Work out the finished part from the listing and answer in its coordinate system (mm). Coordinates: 2 decimals unless noted, no trailing zeros.
1. The part is cut by section A-A, the plane z = -1.6. Count the separate pieces of the cut face and the enclosed holes in it, then the cut area to 3 significant figures.
2. Flat-ended cylindrical pins translate along their axes: pin 1 Ø10.5 at (x, y) = (60, 0) entering from +Z; pin 2 Ø1 at (x, z) = (-4.5, -0.5) entering from +Y; pin 3 Ø5 at (x, y) = (-32.63, 15.21) entering from -Z; pin 4 Ø1 at (x, z) = (46, -2) entering from -Y. Find the tip coordinate at first contact, or state that the pin passes through.
3. Find the intervals of material crossed by probe 1 along X at (y, z) = (-2.5, -2); probe 2 along X at (y, z) = (3.5, -0.2); probe 3 along Y at (x, z) = (-33, -1.8), in increasing order.
```python
from build123d import *

# Parameters (mm, degrees)
EXTRUDE_1_DEPTH     = 3
SKETCH_2_R          = 4
SKETCH_2_R_2        = 6
CUT_EXTRUDE_1_DEPTH = 5
CUT_EXTRUDE_START   = -10
CUT_EXTRUDE_2_DEPTH = 10
FILLET_1_R          = 2
EXTRUDE_START       = -3
EXTRUDE_2_DEPTH     = 3
FILLET_3_R          = 2
EXTRUDE_START_2     = 0.25
SKETCH_6_R          = 8
EXTRUDE_3_DEPTH     = 0.25
SKETCH_7_R          = 7
SKETCH_7_R_2        = 5
CUT_EXTRUDE_4_DEPTH = 1
SKETCH_4_R          = 86.502313977
CUT_EXTRUDE_5_DEPTH = 11
FILLET_5_R          = 5
FILLET_6_R          = 1
SKETCH_8_R          = 14.07038583
CUT_EXTRUDE_6_DEPTH = 0.25


# Some blends are built 0.0001 mm under size
with BuildPart() as part:
    # 草图1 → 凸台-拉伸1 (new body)
    with BuildSketch(Plane.XY):
        with BuildLine():
            Line((60.533333333, -7.982202425), (0.8, -11.973303638))
            ThreePointArc((0.8, -11.973303638), (-2.939445104, -11.634417153), (-6.391104371, -10.156465178))
            Line((-6.391104371, -10.156465178), (-36.621520565, 8.866466686))
            ThreePointArc((-36.621520565, 8.866466686), (-39.424388736, 18.383894386), (-30.331967202, 22.3544574))
            Line((-30.331967202, 22.3544574), (-0.067539503, 12.626398572))
            ThreePointArc((-0.067539503, 12.626398572), (2.297970236, 12.022555106), (4.719428847, 11.711425782))
            Line((4.719428847, 11.711425782), (60.533333333, 7.982202425))
            ThreePointArc((60.533333333, 7.982202425), (68, 0), (60.533333333, -7.982202425))
        make_face()
    extrude(amount=EXTRUDE_1_DEPTH)

    # 草图2 → 切除-拉伸1 (cut)
    with BuildSketch(Plane.XY.offset(3)):
        with Locations((-32.627080333, 15.214257423)):
            Circle(SKETCH_2_R)
        with Locations((60, 0)):
            Circle(SKETCH_2_R)
        Circle(SKETCH_2_R_2)
    extrude(amount=-CUT_EXTRUDE_1_DEPTH, mode=Mode.SUBTRACT)

    # 草图3 → 切除-拉伸2 (cut)
    with BuildSketch(Plane.XY.offset(3).offset(CUT_EXTRUDE_START)):
        with BuildLine():
            Line((28.230392562, -4.127155499), (29.041000535, 4.072994476))
            Line((29.041000535, 4.072994476), (10.769185117, 5.293831496))
            ThreePointArc((10.769185117, 5.293831496), (11.688246691, 2.71751528), (12, 0))
            ThreePointArc((12, 0), (11.688246691, -2.71751528), (10.769185117, -5.293831496))
            Line((10.769185117, -5.293831496), (28.230392562, -4.127155499))
        make_face()
        with BuildLine():
            ThreePointArc((-11.991309043, 0.456626154), (-10.875693444, 5.071419141), (-8.057660805, 8.892362024))
            Line((-8.057660805, 8.892362024), (-24.425138032, 14.153448832))
            ThreePointArc((-24.425138032, 14.153448832), (-25.131680833, 11.719095235), (-26.54234692, 9.613079718))
            Line((-26.54234692, 9.613079718), (-11.991309043, 0.456626154))
        make_face()
        with BuildLine():
            Line((52.404599069, 2.511948386), (35.030683756, 3.672791932))
            Line((35.030683756, 3.672791932), (34.299724154, -3.721631224))
            Line((34.299724154, -3.721631224), (52.404599069, -2.511948386))
            ThreePointArc((52.404599069, -2.511948386), (52, 0), (52.404599069, 2.511948386))
        make_face()
    extrude(amount=CUT_EXTRUDE_2_DEPTH, mode=Mode.SUBTRACT)

    # 圆角1
    fillet_1_edges = [part.edges().sort_by_distance(p)[0] for p in [
        (52.404599069, 2.511948386, 1.5),
        (52.404599069, -2.511948386, 1.5),
        (34.299724154, -3.721631224, 1.5),
        (35.030683756, 3.672791932, 1.5),
        (-26.54234692, 9.613079718, 1.5),
        (-24.425138032, 14.153448832, 1.5),
        (-8.057660805, 8.892362024, 1.5),
        (-11.991309043, 0.456626154, 1.5),
        (10.769185117, -5.293831496, 1.5),
        (10.769185117, 5.293831496, 1.5),
        (29.041000535, 4.072994476, 1.5),
        (28.230392562, -4.127155499, 1.5),
    ]]
    fillet(fillet_1_edges, radius=FILLET_1_R)

    # 草图5 → 凸台-拉伸2 (add)
    with BuildSketch(Plane.XY.offset(3).offset(EXTRUDE_START)):
        with BuildLine():
            Line((-24.540394024, 20.492840682), (-0.067539503, 12.626398572))
            ThreePointArc((-0.067539503, 12.626398572), (29.515306686, 4.823317954), (59.944614351, 7.999808275))
            ThreePointArc((59.944614351, 7.999808275), (62.829825639, 7.482786036), (65.335143615, 5.96122828))
            ThreePointArc((65.335143615, 5.96122828), (18.485789408, 1.404205763), (-24.540394024, 20.492840682))
        make_face()
    extrude(amount=EXTRUDE_2_DEPTH)

    # 圆角3
    # the kernel refuses this fillet: 2 mm, written as the material it adds along each edge
    with BuildSketch(Plane(origin=(51.482720464, 2.033055033, 0), x_dir=(-0.982319810641478, -0.18721054890494518, 0), z_dir=(0, 0, 1))) as fillet_3_piece_1:
        with BuildLine():
            CenterArc((1.886422925, 1.999898233), FILLET_3_R, 170.841064361, 98.580936146)
            Line((-0.088078274, 2.318245549), (-0.285528394, 2.350080281))
            ThreePointArc((-0.285528394, 2.350080281), (-0.438383872, 1.623834826), (-0.169045436, -0.106881432))
            Line((-0.169045436, -0.106881432), (0.002017565, -0.199989823))
            ThreePointArc((0.002017565, -0.199989823), (0.933123639, -0.195293287), (1.864229714, -0.199989823))
            Line((1.864229714, -0.199989823), (1.866247279, 0))
        make_face()
    extrude(amount=3)
    with BuildSketch(Plane(origin=(34.690308342, 0.229537561, 3), x_dir=(-0.09837334507512366, -0.995149579198389, 0), z_dir=(0, 0, -1))) as fillet_3_piece_2:
        with BuildLine():
            CenterArc((1.767742063, -1.99371148), FILLET_3_R, 94.544757631, 77.838582335)
            Line((-0.214612021, -1.728622274), (-0.254259103, -1.72332049))
            ThreePointArc((-0.254259103, -1.72332049), (-0.142932142, -0.859888079), (-0.039739887, 0.004554272))
            Line((-0.039739887, 0.004554272), (0, 0.04))
            ThreePointArc((0, 0.04), (0.8046332, 0.04), (1.606096886, 0.03987423))
            Line((1.606096886, 0.03987423), (1.6092664, 0))
        make_face()
    extrude(amount=3)
    with BuildSketch(Plane(origin=(28.671165111, 0.331721205, 3), x_dir=(-0.9981625762582289, 0.060592667522857975, 0), z_dir=(0, 0, -1))) as fillet_3_piece_3:
        with BuildLine():
            CenterArc((2.077274931, -1.999876599), FILLET_3_R, 90.636478793, 91.535197335)
            Line((0.078711388, -2.075664247), (0.038740118, -2.07718))
            Line((0.038740118, -2.07718), (-0.039971271, -0.001515753))
            Line((-0.039971271, -0.001515753), (0.000444337, 0.039997532))
            ThreePointArc((0.000444337, 0.039997532), (1.027529043, 0.034292711), (2.05461375, 0.039997532))
            Line((2.05461375, 0.039997532), (2.055058086, 0))
        make_face()
    extrude(amount=3)
    with BuildSketch(Plane(origin=(11.680363127, 2.768333075, 0), x_dir=(0.12170231269855974, -0.9925666461673099, 0), z_dir=(0, 0, 1))) as fillet_3_piece_4:
        with BuildLine():
            CenterArc((2.831331682, 1.988408565), FILLET_3_R, 161.255131194, 102.573219996)
            Line((0.937413857, 2.631117886), (0.748022074, 2.695388818))
            ThreePointArc((0.748022074, 2.695388818), (0.290238781, 1.379143519), (-0.187364942, 0.069959836))
            Line((-0.187364942, 0.069959836), (0.008579816, -0.199815882))
            ThreePointArc((0.008579816, -0.199815882), (0.136091641, -0.190622784), (2.594815369, -0.198840857))
            Line((2.594815369, -0.198840857), (2.616316852, 0))
        make_face()
    extrude(amount=3)

    # 草图6 → 凸台-拉伸3 (add)
    with BuildSketch(Plane(origin=(0, 0, 0), x_dir=(-1, 0, 0), z_dir=(0, 0, -1)).offset(EXTRUDE_START_2)):
        with Locations((-60, 0)):
            Circle(SKETCH_6_R)
    extrude(amount=-EXTRUDE_3_DEPTH)

    # 草图7 → 切除-拉伸4 (cut)
    with BuildSketch(Plane(origin=(0, 0, -0.25), x_dir=(-1, 0, 0), z_dir=(0, 0, -1))):
        with Locations((-60, 0)):
            Circle(SKETCH_7_R)
        with Locations((-60, 0)):
            Circle(SKETCH_7_R_2, mode=Mode.SUBTRACT)
    extrude(amount=-CUT_EXTRUDE_4_DEPTH, mode=Mode.SUBTRACT)

    # 草图4 → 切除-拉伸5 (cut)
    with BuildSketch(Plane.XY.offset(3)):
        with Locations((36.403919295, 91.050979361)):
            Circle(SKETCH_4_R)
    extrude(amount=-CUT_EXTRUDE_5_DEPTH, mode=Mode.SUBTRACT)

    # 圆角5
    fillet_5_edges = [part.edges().sort_by_distance(p)[0] for p in [
        (60.533333333, 7.982202425, 1.375),
        (-0.158941589, 12.65577844, 1.5),
    ]]
    fillet(fillet_5_edges, radius=FILLET_5_R)

    # 圆角6
    fillet_6_edges = [part.edges().sort_by_distance(p)[0] for p in [
        (67, 0, 0.75),
        (65, 0, 0.75),
    ]]
    fillet(fillet_6_edges, radius=FILLET_6_R - 0.0001)  # a hair under: the kernel refuses the full size

    # 草图8 → 切除-拉伸6 (cut)
    with BuildSketch(Plane(origin=(0, 0, -0.25), x_dir=(-1, 0, 0), z_dir=(0, 0, -1))):
        with Locations((-60, 0)):
            Circle(SKETCH_8_R)
    extrude(amount=-CUT_EXTRUDE_6_DEPTH, mode=Mode.SUBTRACT)


with BuildPart() as body_2:
    # 镜向1: mirrored copy
    add(part.part.mirror(Plane.XY))


solid = body_2.part
```
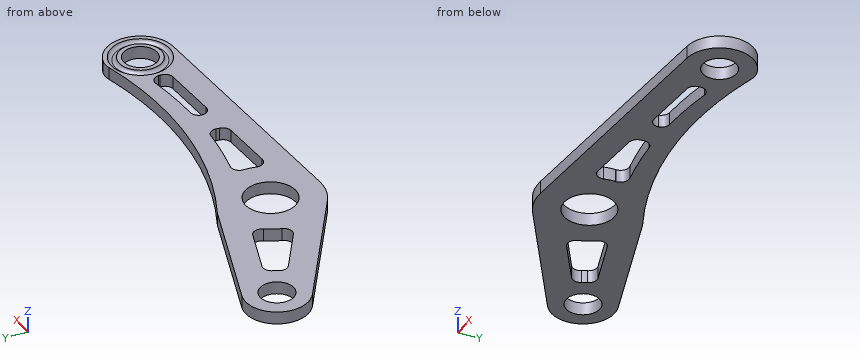
Geometry says:
1. separate pieces: 1
1. enclosed holes: 6
1. area: 1,410 mm2
2. pin 1: stops at z = 0
2. pin 2: stops at y = 14.21
2. pin 3: passes through
2. pin 4: stops at y = -8.99
3. probe 1: x = -18.56 to -5.45, 5.45 to 11.74, 28.39 to 34.75, 50.82 to 56.88, 63.12 to 67.6
3. probe 2: x = -28.09 to -16.83, -11.48 to -4.87, 4.87 to 54.06, 56.28 to 58.06, 61.94 to 63.72, 65.94 to 67.19
3. probe 3: y = 6.59 to 11.23, 19.2 to 22.7
